CAD build for the part. Positions are in the model's coordinates, mm. Face numbers are marked on the shaded views. Round coordinates to 2 decimals unless told otherwise and drop trailing zeros. Loops run counter-clockwise (first coordinate to the right, second up) from the corner with the lowest first, then second, coordinate; pieces in that order, holes last.
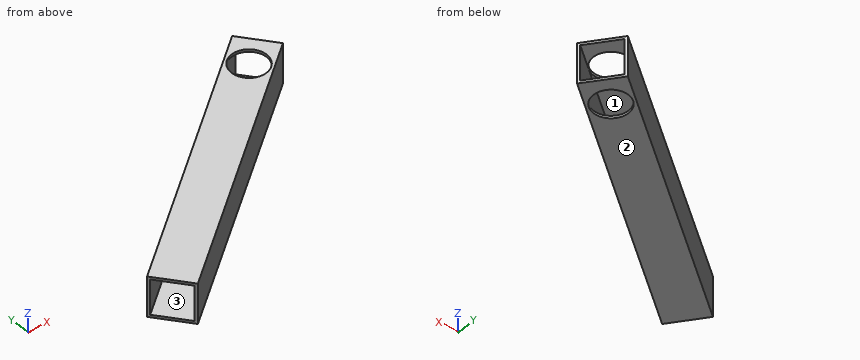
Autodesk Inventor part; units mm, degrees
ref_plane "YZ Plane" through (0, 0, 0) normal (1, 0, 0) x (0, 1, 0)
ref_plane "XZ Plane" through (0, 0, 0) normal (0, 1, 0) x (-1, 0, 0)
ref_plane "XY Plane" through (0, 0, 0) normal (0, 0, 1) x (1, 0, 0)
sketch "Sketch1" plane through (0, 0, 0) normal (0, 0, 1) x (1, 0, 0)
  line L0 (-42.6455, -61.8334) -> (-57.8855, -41.5134)
  line L1 (-57.8855, -41.5134) -> (94.5145, 72.7866)
  line L2 (94.5145, 72.7866) -> (109.7545, 52.4666)
  line L3 (109.7545, 52.4666) -> (-42.6455, -61.8334)
  point P0 (0, 0)
  dimension "d0" = 25.4
  dimension "d1" = 190.5
extrude "Extrusion1" add sketch "Sketch1" along normal blind 25.4
shell "Shell1" thickness 1.5875 removed faces 2 at (-47.7255, -55.0601, 8.4667) at (99.5945, 66.0133, 16.9333)
sketch "Sketch2" plane through (0, 0, 25.4) normal (0, 0, 1) x (1, 0, 0)
  line L0 (109.7545, 52.4666) -> (-42.6455, -61.8334)
  line L1 (94.5145, 72.7866) -> (109.7545, 52.4666)
  circle A0 centre (86.8945, 51.1966) radius 11.1125
  point P0 (0, 0)
  dimension "d5" = 22.225
  dimension "d6" = 12.7
  dimension "d7" = 19.05
extrude "Extrusion2" cut sketch "Sketch2" against normal through all
properties part number "Shovel_RollerMount" material "Aluminum-6061"
Item 1: Wall check: L1, parallel to Z at x = -12, y = -21.5; L2, parallel to Y at x = 40, z = 19.75; L3, parallel to X at y = 13, z = 8. Give the ranges that are in metal, low to high.
Verdict:
L1: z = 0 to 1.59, 23.81 to 25.4
L2: y = 0.15 to 2.14, 29.92 to 31.9
L3: x = 14.8 to 17.44, 54.49 to 57.13
Item 2: Cut at B-B (x = 87). List the corners of the cut face in (y, z).
Verdict:
outline: (35.4, 0) - (40.08, 0) - (40.08, 1.59) - (37.39, 1.59) - (37.39, 23.81) - (40.08, 23.81) - (40.08, 25.4) - (35.4, 25.4) - close; (62.31, 0) - (67.15, 0) - (67.15, 25.4) - (62.31, 25.4) - (62.31, 23.81) - (65.17, 23.81) - (65.17, 1.59) - (62.31, 1.59) - close
Item 3: Cut at D-D (y = -52). List the corners of the cut face in (x, z), plus the area to 3 significant figures.
Verdict:
outline: (-50.02, 0) - (-29.53, 0) - (-29.53, 25.4) - (-50.02, 25.4) - (-50.02, 23.81) - (-32.18, 23.81) - (-32.18, 1.59) - (-50.02, 1.59) - close
area: 124 mm2
Item 4: Mould opens along X. For the marked faces 1, 2 and 3 say: released by +X, released by -X, zero draft, split by the parting line, or undercut.
Verdict:
face 1: undercut
face 2: zero draft
face 3: undercut
Item 5: Cut at A-A (z = 6.75). List the corners of the cut face in (x, y), plus the area to 3 significant figures.
Verdict:
outline: (-57.89, -41.51) - (-56.93, -42.78) - (95.47, 71.52) - (94.51, 72.79) - close; (-43.6, -60.56) - (-42.65, -61.83) - (109.75, 52.47) - (108.8, 53.74) - close
area: 605 mm2
Item 6: Cut at C-C (y = -31). List the corners of the cut face in (x, z), plus the area to 3 significant figures.
Verdict:
outline: (-43.87, 0) - (-1.53, 0) - (-1.53, 25.4) - (-43.87, 25.4) - close; hole (-41.22, 1.59) - (-4.18, 1.59) - (-4.18, 23.81) - (-41.22, 23.81) - close
area: 252 mm2
Item 7: Flat gauge pins, fed straight in: P1, Ø3, axis at x = 28.5, z = 15.5, coming from the -Y side; P2, Ø8, axis at y = 29, z = 16.5, coming from the -X side; P3, Ø1.5, axis at y = -19.5, z = 3, coming from the -X side. Where does each tip first touch, or does it go through?
Verdict:
P1: stops at y = -9.6
P2: stops at x = 30.8
P3: stops at x = -29.53
